```python
from build123d import *

# Parameters (mm, degrees)
SKETCH2_R           = 23.335
SKETCH2_R_2         = 13.335
BOSS_EXTRUDE1_DEPTH = 3.5
SKETCH3_R           = 2.5
SKETCH6_R           = 23.335
SKETCH6_R_2         = 13.335
BOSS_EXTRUDE2_DEPTH = 12.5
SKETCH4_R           = 1.625
CUT_EXTRUDE1_DEPTH  = 17
SKETCH10_W          = 12.5
SKETCH10_H          = 11
CUT_EXTRUDE3_DEPTH  = 20
CUT_EXTRUDE4_DEPTH  = 24.335
CUT_EXTRUDE7_START  = 11.779632
SKETCH14_W          = 12.5
SKETCH14_H          = 1
CUT_EXTRUDE7_DEPTH  = 8.220368
SKETCH16_W          = 4
SKETCH16_H          = 6
CUT_EXTRUDE9_DEPTH  = 4.335000135
CUT_EXTRUDE10_DEPTH = 32.876202934
CUT_EXTRUDE11_DEPTH = 12


with BuildPart() as part:
    # Sketch2 → Boss-Extrude1 (new body)
    with BuildSketch(Plane.XY):
        Circle(SKETCH2_R)
        Circle(SKETCH2_R_2, mode=Mode.SUBTRACT)
    extrude(amount=BOSS_EXTRUDE1_DEPTH)

    # Sketch3 → Cut-Revolve1 (revolve, cut)
    with BuildSketch(Plane(origin=(0, 0, 0), x_dir=(1, 0, 0), z_dir=(0, 1, 0))):
        with Locations((-23.335, -3.5)):
            Circle(SKETCH3_R)
    revolve(axis=Axis((0, 0, 3.5), (0, 0, -1)), mode=Mode.SUBTRACT)

    # Sketch6 → Boss-Extrude2 (add)
    with BuildSketch(Plane(origin=(0, 0, 0), x_dir=(-1, 0, 0), z_dir=(0, 0, -1))):
        Circle(SKETCH6_R)
        Circle(SKETCH6_R_2, mode=Mode.SUBTRACT)
    extrude(amount=BOSS_EXTRUDE2_DEPTH)

    # Sketch4 → Cut-Extrude1 (cut, through all)
    with BuildSketch(Plane(origin=(0, 0, 3.5), x_dir=(-1, 0, 0), z_dir=(0, 0, -1))):
        with Locations((8.5425, 14.796044024)):
            Circle(SKETCH4_R)
        with Locations((-8.5425, 14.796044024)):
            Circle(SKETCH4_R)
        with Locations((-17.085, 0)):
            Circle(SKETCH4_R)
        with Locations((-8.5425, -14.796044024)):
            Circle(SKETCH4_R)
        with Locations((8.5425, -14.796044024)):
            Circle(SKETCH4_R)
        with Locations((17.085, 0)):
            Circle(SKETCH4_R)
    extrude(amount=CUT_EXTRUDE1_DEPTH, mode=Mode.SUBTRACT)

    # Sketch10 → Cut-Extrude3 (cut)
    with BuildSketch(Plane(origin=(0, 0, 0), x_dir=(1, 0, 0), z_dir=(0, 1, 0))):
        with Locations((0, 6)):
            Rectangle(SKETCH10_W, SKETCH10_H)
        with BuildLine():
            ThreePointArc((5.5, 6.5), (4.5, 7.5), (3.5, 6.5))
            Line((3.5, 6.5), (3.5, 5.5))
            ThreePointArc((3.5, 5.5), (4.5, 4.5), (5.5, 5.5))
            Line((5.5, 5.5), (5.5, 6.5))
        make_face(mode=Mode.SUBTRACT)
        with BuildLine():
            ThreePointArc((-5.5, 5.5), (-4.5, 4.5), (-3.5, 5.5))
            Line((-3.5, 5.5), (-3.5, 6.5))
            ThreePointArc((-3.5, 6.5), (-4.5, 7.5), (-5.5, 6.5))
            Line((-5.5, 6.5), (-5.5, 5.5))
        make_face(mode=Mode.SUBTRACT)
        with BuildLine():
            ThreePointArc((-2, 5.5), (0, 3.5), (2, 5.5))
            Line((2, 5.5), (2, 6.5))
            ThreePointArc((2, 6.5), (0, 8.5), (-2, 6.5))
            Line((-2, 6.5), (-2, 5.5))
        make_face(mode=Mode.SUBTRACT)
        with BuildLine():
            Line((5.5, 5.5), (5.5, 6.5))
            ThreePointArc((5.5, 6.5), (4.5, 7.5), (3.5, 6.5))
            Line((3.5, 6.5), (3.5, 5.5))
            ThreePointArc((3.5, 5.5), (4.5, 4.5), (5.5, 5.5))
        make_face()
        with BuildLine():
            Line((-2, 6.5), (-2, 5.5))
            ThreePointArc((-2, 5.5), (0, 3.5), (2, 5.5))
            Line((2, 5.5), (2, 6.5))
            ThreePointArc((2, 6.5), (0, 8.5), (-2, 6.5))
        make_face()
        with BuildLine():
            Line((-5.5, 6.5), (-5.5, 5.5))
            ThreePointArc((-5.5, 5.5), (-4.5, 4.5), (-3.5, 5.5))
            Line((-3.5, 5.5), (-3.5, 6.5))
            ThreePointArc((-3.5, 6.5), (-4.5, 7.5), (-5.5, 6.5))
        make_face()
    extrude(amount=CUT_EXTRUDE3_DEPTH, mode=Mode.SUBTRACT)

    # Sketch10<3> → Cut-Extrude4 (cut, through all)
    with BuildSketch(Plane(origin=(0, 0, 0), x_dir=(1, 0, 0), z_dir=(0, 1, 0))):
        with BuildLine():
            Line((5.5, 5.5), (5.5, 6.5))
            ThreePointArc((5.5, 6.5), (4.5, 7.5), (3.5, 6.5))
            Line((3.5, 6.5), (3.5, 5.5))
            ThreePointArc((3.5, 5.5), (4.5, 4.5), (5.5, 5.5))
        make_face()
        with BuildLine():
            Line((-2, 6.5), (-2, 5.5))
            ThreePointArc((-2, 5.5), (0, 3.5), (2, 5.5))
            Line((2, 5.5), (2, 6.5))
            ThreePointArc((2, 6.5), (0, 8.5), (-2, 6.5))
        make_face()
        with BuildLine():
            Line((-5.5, 6.5), (-5.5, 5.5))
            ThreePointArc((-5.5, 5.5), (-4.5, 4.5), (-3.5, 5.5))
            Line((-3.5, 5.5), (-3.5, 6.5))
            ThreePointArc((-3.5, 6.5), (-4.5, 7.5), (-5.5, 6.5))
        make_face()
    extrude(amount=CUT_EXTRUDE4_DEPTH, mode=Mode.SUBTRACT)

    # Sketch14 → Cut-Extrude7 (cut)
    with BuildSketch(Plane(origin=(0, 0, 0), x_dir=(1, 0, 0), z_dir=(0, 1, 0)).offset(CUT_EXTRUDE7_START)):
        with Locations((0, 12)):
            Rectangle(SKETCH14_W, SKETCH14_H)
    extrude(amount=CUT_EXTRUDE7_DEPTH, mode=Mode.SUBTRACT)

    # Sketch16 → Cut-Extrude9 (cut, through all)
    with BuildSketch(Plane.XZ.offset(-20)):
        with Locations((0, -9.5)):
            Rectangle(SKETCH16_W, SKETCH16_H)
    extrude(amount=-CUT_EXTRUDE9_DEPTH, mode=Mode.SUBTRACT)

    # Sketch17 → Cut-Extrude10 (cut, through all)
    with BuildSketch(Plane(origin=(0, 0, 0), x_dir=(0, 0, -1), z_dir=(-0.866025404, -0.5, 0))):
        with BuildLine():
            Line((10.25, 2.5), (10.25, -2.5))
            ThreePointArc((10.25, -2.5), (8.25, -4.5), (6.25, -2.5))
            Line((6.25, -2.5), (6.25, 2.5))
            ThreePointArc((6.25, 2.5), (8.25, 4.5), (10.25, 2.5))
        make_face()
    extrude(amount=CUT_EXTRUDE10_DEPTH, mode=Mode.SUBTRACT)

    # Sketch18 → Cut-Extrude11 (cut)
    with BuildSketch(Plane(origin=(0, 0, -12.5), x_dir=(-1, 0, 0), z_dir=(0, 0, -1))):
        with BuildLine():
            Line((-6.25, 11.779631785), (-6.25, 18.998355192))
            ThreePointArc((-6.25, 18.998355192), (0, 20), (6.25, 18.998355192))
            Line((6.25, 18.998355192), (6.25, 11.779631785))
            ThreePointArc((6.25, 11.779631785), (10.692886041, 11.676726964), (12.177094021, 15.865635229))
            ThreePointArc((12.177094021, 15.865635229), (17.337033787, 9.971321851), (19.837129792, 2.547210554))
            ThreePointArc((19.837129792, 2.547210554), (13.335, 0), (19.837129792, -2.547210554))
            ThreePointArc((19.837129792, -2.547210554), (17.320508076, -10), (12.124513945, -15.905853061))
            ThreePointArc((12.124513945, -15.905853061), (6.6675, -11.548448759), (7.712615847, -18.453063615))
            ThreePointArc((7.712615847, -18.453063615), (0, -20), (-7.712615847, -18.453063615))
            ThreePointArc((-7.712615847, -18.453063615), (-6.6675, -11.548448759), (-12.124513945, -15.905853061))
            ThreePointArc((-12.124513945, -15.905853061), (-17.320508076, -10), (-19.837129792, -2.547210554))
            ThreePointArc((-19.837129792, -2.547210554), (-13.335, 0), (-19.837129792, 2.547210554))
            ThreePointArc((-19.837129792, 2.547210554), (-17.337033787, 9.971321851), (-12.177094021, 15.865635229))
            ThreePointArc((-12.177094021, 15.865635229), (-10.692886041, 11.676726964), (-6.25, 11.779631785))
        make_face()
    extrude(amount=-CUT_EXTRUDE11_DEPTH, mode=Mode.SUBTRACT)


solid = part.part
```
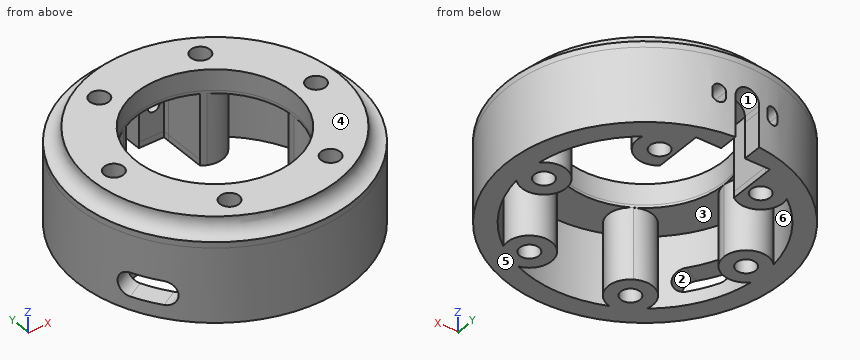
The model under review builds one solid part; all positions refer to its coordinate system, in mm. Face numbers are marked on the shaded views. A direction names the side the tool comes from. Round coordinates to 2 decimals unless told otherwise and drop trailing zeros.
(1) Machinability: for the marked faces 1, 2, 3 and 4, which of the approach directions +Z, -Z, +X, -X, +Y, -Y give a long, thin tool a straight path to every point of the face, cutting with its end or side? Answer none if there is none.
(2) We need section A-A on z = -8.25. Give the number of separate pieces and of enclosed holes in the cut face, and give its area (3 significant figures).
(3) Wall thickness on L1, parallel to X at y = 0, z = -1 (3 decimals); L2, parallel to X at y = 12, z = -7.75; L3, parallel to Y at x = -8, z = -7.5: over which ranges is each line inside the solid? List them lowest first.
(4) Mouldability with a two-part tool opening along Y and no side actions: class the marked faces 5 and 6 as +Y half, -Y half, draft (parallel to the pull), parting line (faces both ways), or undercut.
(5) Insertion check: pin 1 (1 mm diameter, centred on x = 4.5, z = -1, fed in from -Y); pin 2 (1.1 mm diameter, centred on y = 19.5, z = -8, fed in from +X); pin 3 (0.8 mm diameter, centred on x = 3.5, z = -12, fed in from -Y). Each pin has a flat end and moves straight along its axis. Give the tip position at first contact, or say it passes through.
Findings below:
1. face 1: -Z, +Y
1. face 2: -X
1. face 3: -Z
1. face 4: +Z, +X, -X, +Y, -Y
2. separate pieces: 2
2. enclosed holes: 6
2. area: 594 mm2
3. L1: x = -23.335 to -18.71, -15.46 to -13.335, 13.335 to 15.46, 18.71 to 23.335
3. L2: x = -20.01 to -16, -11.1 to -6.25, 6.25 to 11.1, 16 to 20.01
3. L3: y = -21.92 to -16.33, -13.26 to -11.09, 11.05 to 13.26, 16.33 to 21.92
4. face 5: draft
4. face 6: undercut
5. pin 1: stops at y = -22.99
5. pin 2: stops at x = 13.62
5. pin 3: stops at y = -23.13
